Verification items for this drawing (mm, ordinates from the low corner). A direction names the side the tool comes from. Round coordinates to 2 decimals unless told otherwise and drop trailing zeros. Loops run counter-clockwise (first coordinate to the right, second up) from the corner with the lowest first, then second, coordinate; pieces in that order, holes last. Notation, with made-up numbers: (-31, 47) -> (8, 47) arc R13 ccw to (8, 60) -> close; hole circle Ø3 at (-7.5, 78.25). An arc over 180 degrees is marked (long way). One line per item, written item: value. Start each with the question number.
1. Cross-section at A-A on x = 60. Count the separate pieces of the cut face and the enclosed holes in it, then the cut area to 3 significant figures.
2. Cross-section at C-C on z = 15.5. Record the cut outline in (x, y) (1 decimal).
3. Release check for a two-part mould opening along Y. For the marked faces 4, 5 and 6 record: +Y half, -Y half, draft (parallel to the pull), parting line (faces both ways), or undercut.
4. Go/stop test with flat-tipped pins: pin 1 (1.6 mm diameter, centred on y = 70.5, z = 23, fed in from -X); pin 2 (19 mm diameter, centred on x = 36.22, y = 67.73, fed in from -Z); pin 3 (3 mm diameter, centred on x = 79.5, y = 62, fed in from +Z). Record where each tip stops, or that it passes through.
5. Cross-section at B-B on y = 60. Record the cut outline in (x, z), then the cut area to 3 significant figures.
6. Set-up check for the marked faces 1, 2 and 3: record each of +Z, -Z, +X, -X, +Y, -Y from which the full face is reachable in a straight line by a thin tool's end or side.
7. Material ranges on L1, parallel to X at y = 63, z = 13 (1 decimal); L2, parallel to Z at x = 46.5, y = 73; L3, parallel to Z at x = 53, y = 52, recorded low to high.
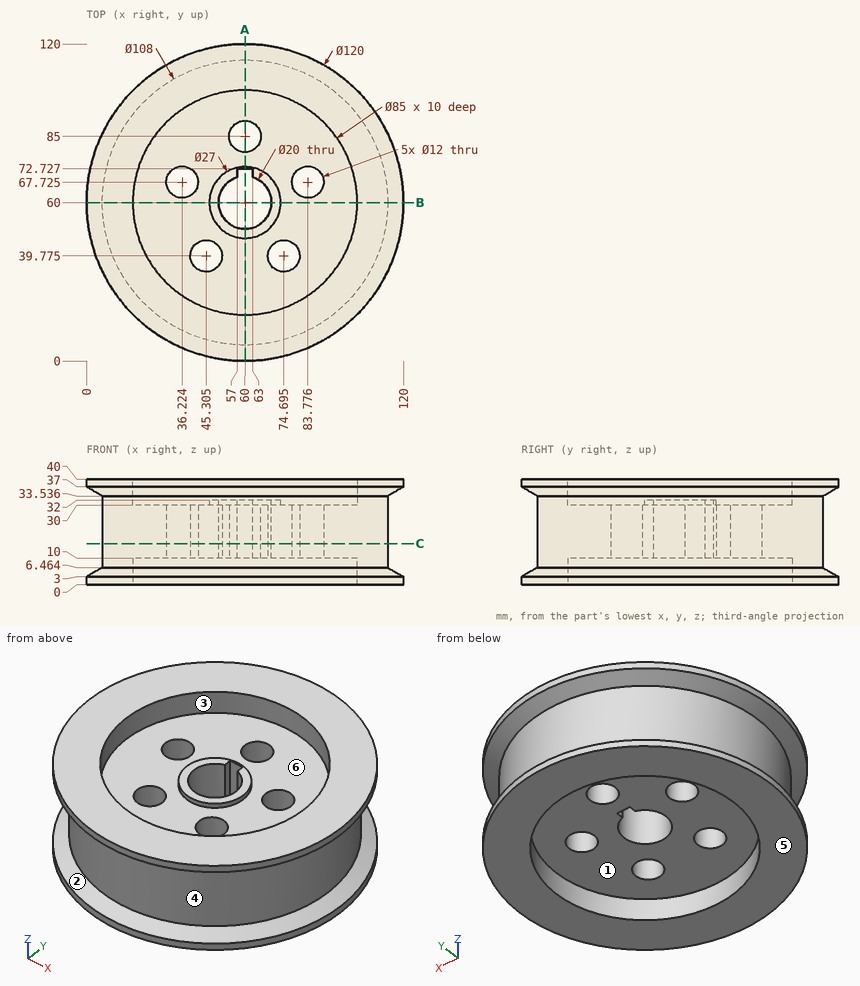
Taken from the geometry:
1. separate pieces: 3
1. enclosed holes: 0
1. area: 2,050 mm2
2. outline: circle Ø108 at (60, 60); hole circle Ø12 at (36.2, 67.7); hole circle Ø12 at (45.3, 39.8); hole circle Ø12 at (60, 85); hole (57, 69.5) arc R10 ccw (long way) to (63, 69.5) -> (63, 72.7) -> (57, 72.7) -> close; hole circle Ø12 at (74.7, 39.8); hole circle Ø12 at (83.8, 67.7)
3. face 4: parting line
3. face 5: draft
3. face 6: undercut
4. pin 1: stops at x = 6.88
4. pin 2: stops at z = 10
4. pin 3: stops at z = 30
5. outline: (0, 0) -> (17.5, 0) -> (17.5, 10) -> (50, 10) -> (50, 32) -> (46.5, 32) -> (46.5, 30) -> (17.5, 30) -> (17.5, 40) -> (0, 40) -> (0, 37) -> (6, 33.54) -> (6, 6.46) -> (0, 3) -> close; (70, 10) -> (102.5, 10) -> (102.5, 0) -> (120, 0) -> (120, 3) -> (114, 6.46) -> (114, 33.54) -> (120, 37) -> (120, 40) -> (102.5, 40) -> (102.5, 30) -> (73.5, 30) -> (73.5, 32) -> (70, 32) -> close
5. area: 2,350 mm2
6. face 1: -Z
6. face 2: none
6. face 3: +Z
7. L1: x = 6.1 to 32.5, 39.9 to 50.5, 69.5 to 80.1, 87.5 to 113.9
7. L2: z = 10 to 30
7. L3: z = 10 to 32
